Geometry: see drawing. Coordinates: mm, zero at the bounding-box minimum. A direction names the side the tool comes from. Coordinates: 2 decimals unless noted, no trailing zeros. Write each loop counter-clockwise with the first axis right and the second up, starting at its lowest first coordinate (ties: lowest second). Pieces come first, ordered by that corner, then holes.
1) Line query: L1, parallel to X at y = 0.8, z = 7; L2, parallel to Z at x = 3.5, y = 0.5; L3, parallel to X at y = 1.1, z = 12.75. Output: solid intervals per line, ascending.
2) Section query C-C (y = 1.5). Output: boundary loops of the cut face in (x, z).
3) Section query A-A (z = 7). Output: boundary loops of the cut face in (x, y).
4) Section query D-D (z = 1.75). Output: boundary loops of the cut face in (x, y).
5) Pin query (flat end, axial travel): pin 1 Ø1.8 at (x, z) = (39.5, 7) entering from -Y; pin 2 Ø0.8 at (x, y) = (38, 1.5) entering from +Z; pin 3 Ø0.8 at (y, z) = (1, 1) entering from +X; pin 4 Ø0.8 at (x, y) = (40, 1) entering from -Z. Return the tip coordinate at first contact, or that it passes through.
6) Set-up query: the marked faces 1, 2, 3 and 4. Return all of +Z, -Z, +X, -X, +Y, -Y with unobstructed straight access to the full face (end or side cutting, diameter ignored); none if empty.
7) Section query B-B (x = 3.5). Output: boundary loops of the cut face in (y, z).
8) Draft query along Z for the marked faces 5, 6 and 7. Return one class per face: pulls with the +Z half, pulls with the -Z half, needs draft (parallel to the pull), parting line crosses it, or undercut.
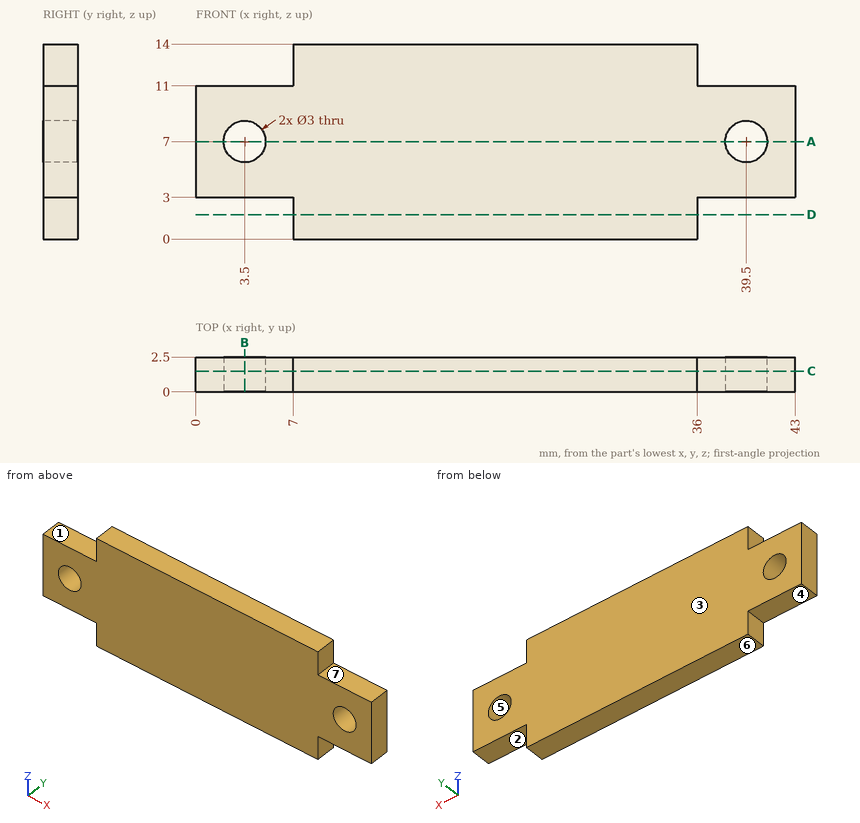
Answer:
1. L1: x = 0 to 2, 5 to 38, 41 to 43
1. L2: z = 3 to 5.5, 8.5 to 11
1. L3: x = 7 to 36
2. outline: (0, 3) - (7, 3) - (7, 0) - (36, 0) - (36, 3) - (43, 3) - (43, 11) - (36, 11) - (36, 14) - (7, 14) - (7, 11) - (0, 11) - close; hole circle Ø3 at (3.5, 7); hole circle Ø3 at (39.5, 7)
3. outline: (0, 0) - (2, 0) - (2, 2.5) - (0, 2.5) - close; (5, 0) - (38, 0) - (38, 2.5) - (5, 2.5) - close; (41, 0) - (43, 0) - (43, 2.5) - (41, 2.5) - close
4. outline: (7, 0) - (36, 0) - (36, 2.5) - (7, 2.5) - close
5. pin 1: passes through
5. pin 2: stops at z = 11
5. pin 3: stops at x = 36
5. pin 4: stops at z = 3
6. face 1: +Z, -X, +Y, -Y
6. face 2: -Z, +X, +Y, -Y
6. face 3: +Z, -Z, +X, -X, +Y
6. face 4: -Z, -X, +Y, -Y
7. outline: (0, 3) - (2.5, 3) - (2.5, 5.5) - (0, 5.5) - close; (0, 8.5) - (2.5, 8.5) - (2.5, 11) - (0, 11) - close
8. face 5: undercut
8. face 6: pulls with the -Z half
8. face 7: pulls with the +Z half
